```python
from build123d import *

# Parameters (mm, degrees)
SALIENTE_EXTRUIR1_DEPTH = 15
CROQUIS2_R              = 5
CORTAR_EXTRUIR1_DEPTH   = 60
CROQUIS3_R              = 4.9
CORTAR_EXTRUIR2_DEPTH   = 60


with BuildPart() as part:
    # Croquis1 → Saliente-Extruir1 (new, symmetric)
    with BuildSketch(Plane.XY):
        Polygon((-13.5, -81), (-13.5, 12.7), (-19.85, 12.7), (-19.85, -87.35), (0, -87.35), (0, -81), align=None)
        Polygon((13.5, -81), (0, -81), (0, -87.35), (19.85, -87.35), (19.85, 12.7), (13.5, 12.7), align=None)
    extrude(amount=SALIENTE_EXTRUIR1_DEPTH, both=True)

    # Croquis2 → Cortar-Extruir1 (cut)
    with BuildSketch(Plane.ZY.offset(19.85)):
        with Locations(Location((0, 0, 0), (0, 0, 270))):
            Circle(CROQUIS2_R)
    extrude(amount=-CORTAR_EXTRUIR1_DEPTH, mode=Mode.SUBTRACT)

    # Croquis3 → Cortar-Extruir2 (cut)
    with BuildSketch(Plane.XZ.offset(87.35)):
        Circle(CROQUIS3_R)
    extrude(amount=-CORTAR_EXTRUIR2_DEPTH, mode=Mode.SUBTRACT)


solid = part.part
```
Verification items for the finished model (mm, model axes). A direction names the side the tool comes from. Round coordinates to 2 decimals unless told otherwise and drop trailing zeros. Write each loop counter-clockwise with the first axis right and the second up, starting at its lowest first coordinate (ties: lowest second). Pieces come first, ordered by that corner, then holes.
1. Section check A-A on y = -58.5. Enter the section's corners in (x, z).
2. Scan lines: L1, parallel to X at y = -1.5, z = 9.75; L2, parallel to Z at x = 0, y = -84; L3, parallel to Z at x = -16, y = 0. Record each from-to range of solid material in increasing order.
3. Section check B-B on x = 0. Enter the section's corners in (y, z).
4. Section check D-D on z = 0. Enter the section's corners in (x, y), plus the area to 3 significant figures.
5. Gauge pin test, flat ends, axial feed: P1, Ø9, axis at y = 0, z = 0, coming from the -X side; P2, Ø3, axis at x = 5, z = -6, coming from the +Y side. Record the tip position at first contact, or that the pin passes through.
6. Section check C-C on y = 0. Enter the section's corners in (x, z).
7. Access from +Z, -Z, +X, -X, +Y, -Y to the whole of each face (thin tool, end or side, straight path). Record for faces 4 (the flat face through (-6, -81, 0)), 5 (the cylindrical face through (-1.062, -84.219, -4.783)).
8. Draft check along X on faces 1 (the flat face through (-19.85, -37, 0)), 2 (the flat face through (13.5, -33, 0)), 3 (the cylindrical face through (-16.72, 1.08, -4.88)). Enter one of: +X half, -X half, draft (parallel to the pull), parting line (faces both ways), or undercut.
Answer:
1. outline: (-19.85, -15) - (-13.5, -15) - (-13.5, 15) - (-19.85, 15) - close; (13.5, -15) - (19.85, -15) - (19.85, 15) - (13.5, 15) - close
2. L1: x = -19.85 to -13.5, 13.5 to 19.85
2. L2: z = -15 to -4.9, 4.9 to 15
2. L3: z = -15 to -5, 5 to 15
3. outline: (-87.35, -15) - (-81, -15) - (-81, -4.9) - (-87.35, -4.9) - close; (-87.35, 4.9) - (-81, 4.9) - (-81, 15) - (-87.35, 15) - close
4. outline: (-19.85, -87.35) - (-4.9, -87.35) - (-4.9, -81) - (-13.5, -81) - (-13.5, -5) - (-19.85, -5) - close; (-19.85, 5) - (-13.5, 5) - (-13.5, 12.7) - (-19.85, 12.7) - close; (4.9, -87.35) - (19.85, -87.35) - (19.85, -5) - (13.5, -5) - (13.5, -81) - (4.9, -81) - close; (13.5, 5) - (19.85, 5) - (19.85, 12.7) - (13.5, 12.7) - close
4. area: 1,250 mm2
5. P1: passes through
5. P2: stops at y = -81
6. outline: (-19.85, -15) - (-13.5, -15) - (-13.5, -5) - (-19.85, -5) - close; (-19.85, 5) - (-13.5, 5) - (-13.5, 15) - (-19.85, 15) - close; (13.5, -15) - (19.85, -15) - (19.85, -5) - (13.5, -5) - close; (13.5, 5) - (19.85, 5) - (19.85, 15) - (13.5, 15) - close
7. face 4: +Z, -Z, +Y
7. face 5: +Y, -Y
8. face 1: -X half
8. face 2: undercut
8. face 3: draft
